Verification items for the finished model (mm, model axes). A direction names the side the tool comes from. Round coordinates to 2 decimals unless told otherwise and drop trailing zeros. Write each loop counter-clockwise with the first axis right and the second up, starting at its lowest first coordinate (ties: lowest second). Pieces come first, ordered by that corner, then holes. Notation, with made-up numbers: (72.5, -2.75) -> (127.5, -2.75) arc R31 cw to (127.5, 35.25) -> close; hole circle Ø5 at (81.5, 69). An arc over 180 degrees is marked (long way). Answer as a JSON object with one key per item and string values. Group by question number.
(1) Scan lines: L1, parallel to Y at x = -88, z = 0.8; L2, parallel to X at y = 315.5, z = 1.55; L3, parallel to Z at x = -84.25, y = 318. Record each from-to range of solid material in increasing order. Write a range as from..to.
(2) Sectioned sample at C-C on z = 12.5. Record the cut outline in (x, y).
(3) Gauge pin test, flat ends, axial feed: pin 1 Ø8 at (x, y) = (-89, 320) entering from +Z; pin 2 Ø3 at (x, z) = (-96, 18.5) entering from +Y; pin 3 Ø8.5 at (y, z) = (315.32, 12.55) entering from +X. Record the tip position at first contact, or that the pin passes through.
(4) Sectioned sample at D-D on z = 8.25. Record the cut outline in (x, y), and give its area (3 significant figures).
(5) Sectioned sample at B-B on y = 323. Record the cut outline in (x, z).
(6) Set-up check for faces 1 (the face through (-81.85, 308.51, 1.52)), 2 (the face through (-95.196, 332.65, 10.638)): record each of +Z, -Z, +X, -X, +Y, -Y from which the full face is reachable in a straight line by a thin tool's end or side.
(7) Sectioned sample at A-A on x = -90. Record the cut outline in (y, z), and give its area (3 significant figures).
(8) Draft check along Y on faces 3 (the face through (-96.56, 333.31, 11.42)), 4 (the face through (-97, 317.4, 10.6)), 5 (the face through (-98, 305.5, 4)). Enter one of: released by +Y, released by -Y, zero draft, split by the parting line, or undercut.
```python
from build123d import *

# Parameters (mm, degrees)
BOSS_EXTRU_1_DEPTH      = 23
ESQUISSE2_R             = 2.6
BOSS_EXTRU_2_DEPTH      = 3
ESQUISSE3_R             = 2.6
ENL_V_MAT_EXTRU_1_DEPTH = 3
ESQUISSE4_R             = 2.6
ENL_V_MAT_EXTRU_2_DEPTH = 3
CONG_1_R                = 10


with BuildPart() as part:
    # Esquisse1 → Boss.-Extru.1 (new body)
    with BuildSketch(Plane.XY):
        Polygon((-100, 325.5), (-100, 305.5), (-97, 305.5), (-97, 325.144463965), (-92.275093963, 344.79877668), (-95.191990577, 345.5), align=None)
    extrude(amount=BOSS_EXTRU_1_DEPTH)

    # Esquisse2 → Boss.-Extru.2 (add)
    with BuildSketch(Plane.XY):
        Polygon((-92.275093963, 344.79877668), (-79, 341.607437837), (-79, 305.5), (-97, 305.5), (-97, 325.144463965), align=None)
        with Locations((-88, 315.5)):
            Circle(ESQUISSE2_R, mode=Mode.SUBTRACT)
        with Locations((-88, 335.5)):
            Circle(ESQUISSE2_R, mode=Mode.SUBTRACT)
    extrude(amount=BOSS_EXTRU_2_DEPTH)

    # Esquisse3 → Enlèv. mat.-Extru.1 (cut)
    with BuildSketch(Plane(origin=(-97, 0, 0), x_dir=(0, 0, -1), z_dir=(1, 0, 0))):
        with Locations((-12.549028202, 315.322231983)):
            Circle(ESQUISSE3_R)
    extrude(amount=-ENL_V_MAT_EXTRU_1_DEPTH, mode=Mode.SUBTRACT)

    # Esquisse4 → Enlèv. mat.-Extru.2 (cut)
    with BuildSketch(Plane(origin=(-165.594765625, 39.809059675, 0), x_dir=(0, 0, -1), z_dir=(0.9722988712431988, -0.23374110673820697, 0))):
        with Locations(Location((-13, 303.571843368, 0), (0, 0, 90))):
            Circle(ESQUISSE4_R)
    extrude(amount=-ENL_V_MAT_EXTRU_2_DEPTH, mode=Mode.SUBTRACT)

    # Congé1
    cong_1_edges = [part.edges().sort_by_distance(p)[0] for p in [
        (-98.5, 305.5, 23),
        (-93.73354227, 345.14938834, 23),
        (-79, 305.5, 1.5),
        (-79, 341.607437837, 1.5),
    ]]
    fillet(cong_1_edges, radius=CONG_1_R)


solid = part.part
```
Computed values:
{
 "1": {"L1": "305.55..312.9, 318.1..332.9, 338.1..343.77", "L2": "-100..-90.6, -85.4..-79", "L3": "0..3"},
 "2": {"outline": "(-100, 305.5) -> (-97, 305.5) -> (-97, 312.72) -> (-100, 312.72) -> close; (-100, 317.92) -> (-97, 317.92) -> (-97, 325.14) -> (-95.23, 332.49) -> (-98.15, 333.19) -> (-100, 325.5) -> close; (-96.96, 338.15) -> (-94.04, 337.45) -> (-92.28, 344.8) -> (-95.19, 345.5) -> close"},
 "3": {"pin 1": "z = 3", "pin 2": "y = 344.63", "pin 3": "x = -97"},
 "4": {"outline": "(-100, 305.5) -> (-97, 305.5) -> (-97, 325.14) -> (-92.28, 344.8) -> (-95.19, 345.5) -> (-100, 325.5) -> close", "area": "121 mm2"},
 "5": {"outline": "(-100, 0) -> (-79, 0) -> (-79, 3) -> (-97, 3) -> (-97, 23) -> (-100, 23) -> close"},
 "6": {"face 1": "+Z, -Z, +X, -Y", "face 2": "+Z, +X, -Y"},
 "7": {"outline": "(305.5, 0) -> (313.84, 0) -> (313.84, 3) -> (305.5, 3) -> close; (317.16, 0) -> (333.84, 0) -> (333.84, 3) -> (317.16, 3) -> close; (337.16, 0) -> (344.25, 0) -> (344.25, 3) -> (337.16, 3) -> close", "area": "96.3 mm2"},
 "8": {"face 3": "undercut", "face 4": "zero draft", "face 5": "released by -Y"}
}
